Check sheet for the modelled part. Datum: model origin and axes. Units: mm. A direction names the side the tool comes from. Give positions to 0.01 mm unless a question says otherwise; leave off trailing zeros. Loops run counter-clockwise (first coordinate to the right, second up) from the corner with the lowest first, then second, coordinate; pieces in that order, holes last. Notation, with made-up numbers: (85.5, 7) - (127.5, 7) arc R20 ccw to (127.5, 46) - close; hole circle Ø10 at (-5, 69.5). An arc over 180 degrees is marked (long way). Use CSV: the item, a comma, the result in double quotes.
from build123d import *

# Parameters (mm, degrees)
F0_R           = 9.525
F1_DEPTH       = 38.1
F4_W           = 7.6494621422
F4_H           = 6.35
F5_DEPTH       = 12.7
F8_D           = 14.732
F8_DEPTH       = 69.85
F8_TIP         = 4.4259393198
F8_ON_F7_D     = 14.732
F8_ON_F7_DEPTH = 69.85
F8_ON_F7_TIP   = 4.4259393198
F9_T4_DEPTH    = 51.5282991577
F9_S5_R        = 9.525
F9_T6_DEPTH    = 28
F9_T10_DEPTH   = 51.965031671
F9_S11_R       = 9.525
F9_T12_DEPTH   = 28
F9_T16_DEPTH   = 51.965031671
F9_S17_R       = 9.525
F9_T18_DEPTH   = 28
F9_T22_DEPTH   = 51.5282991577
F9_S23_R       = 9.525
F9_T24_DEPTH   = 28


# Not quite as in the source:
# - a fillet or chamfer that OpenCascade refuses, or shapes differently, is made with other operations: its cross-section is extruded or revolved along the edge and cut away or added
# - a feature of the source that left no trace in its solid (it failed there, or was rolled back) is left out


with BuildPart() as f1:
    # F0 (on Top) → F1 (new body, symmetric)
    with BuildSketch(Plane.XY):
        with Locations((-15.875, 0)):
            Circle(F0_R)
    extrude(amount=F1_DEPTH, both=True)



with BuildPart() as f1b:
    # F0 (on Top) → F1, piece 2 (new body, symmetric)
    with BuildSketch(Plane.XY):
        with Locations((15.875, 0)):
            Circle(F0_R)
    extrude(amount=F1_DEPTH, both=True)


with BuildPart() as f1_1:
    add(f1.part)

    add(f1b.part)  # F5 merges F1b
    # F4 (on Top) → F5 (join, symmetric)
    with BuildSketch(Plane.XY):
        with Locations((-3.8247310711, 3.175)):
            Rectangle(F4_W, F4_H)
        Polygon((7.4973143637, 0), (0, 0), (0, -6.35), (7.6071062533, -6.35), align=None)
        Polygon((0, 6.35), (0, 0), (7.4973143637, 0), (7.6071062533, 6.35), align=None)
        with Locations((-3.8247310711, -3.175)):
            Rectangle(F4_W, F4_H)
    extrude(amount=F5_DEPTH, both=True)

    # F8
    with Locations(Plane.XY.offset(38.1)):
        with Locations((-15.875, 0)):
            Hole(F8_D / 2, depth=F8_DEPTH)
            with Locations((0, 0, -(F8_DEPTH + F8_TIP / 2))):  # 118° drill point
                Cone(0, F8_D / 2, F8_TIP, mode=Mode.SUBTRACT)

    # F8 on F7
    with Locations(Plane.XY.offset(38.1)):
        with Locations((15.875, 0)):
            Hole(F8_ON_F7_D / 2, depth=F8_ON_F7_DEPTH)
            with Locations((0, 0, -(F8_ON_F7_DEPTH + F8_ON_F7_TIP / 2))):  # 118° drill point
                Cone(0, F8_ON_F7_D / 2, F8_ON_F7_TIP, mode=Mode.SUBTRACT)

    # F9: chamfer of 5.08 on 4 edges, made by hand


with BuildPart() as f9_tool2:
    # F9_s3 → F9_t4 (new body)
    with BuildSketch(Plane.XY.offset(25.7641495789)):
        Polygon((-7.6494621422, -1.27), (-2.5694621422, -6.35), (-7.6494621422, -6.35), align=None)
    extrude(amount=-F9_T4_DEPTH)

    # F9_s5 → F9_t6 (cut, symmetric)
    with BuildSketch(Plane.XY):
        with Locations((-15.875, 0)):
            Circle(F9_S5_R)
    extrude(amount=F9_T6_DEPTH, both=True, mode=Mode.SUBTRACT)


with BuildPart() as f1_2:
    add(f1_1.part)

    # F9_t1: cut F9_tool2
    add(f9_tool2.part, mode=Mode.SUBTRACT)


with BuildPart() as f9_tool8:
    # F9_s9 → F9_t10 (new body)
    with BuildSketch(Plane.XY.offset(25.9825158355)):
        Polygon((7.5177543218, -1.1821796141), (2.438513475, -6.35), (7.6071062533, -6.35), align=None)
    extrude(amount=-F9_T10_DEPTH)

    # F9_s11 → F9_t12 (cut, symmetric)
    with BuildSketch(Plane.XY):
        with Locations((15.875, 0)):
            Circle(F9_S11_R)
    extrude(amount=F9_T12_DEPTH, both=True, mode=Mode.SUBTRACT)


with BuildPart() as f1_3:
    add(f1_2.part)

    # F9_t7: cut F9_tool8
    add(f9_tool8.part, mode=Mode.SUBTRACT)


with BuildPart() as f9_tool14:
    # F9_s15 → F9_t16 (new body)
    with BuildSketch(Plane.XY.offset(-25.9825158355)):
        Polygon((7.5177543218, 1.1821796141), (2.438513475, 6.35), (7.6071062533, 6.35), align=None)
    extrude(amount=F9_T16_DEPTH)

    # F9_s17 → F9_t18 (cut, symmetric)
    with BuildSketch(Plane.XY):
        with Locations((15.875, 0)):
            Circle(F9_S17_R)
    extrude(amount=F9_T18_DEPTH, both=True, mode=Mode.SUBTRACT)


with BuildPart() as f1_4:
    add(f1_3.part)

    # F9_t13: cut F9_tool14
    add(f9_tool14.part, mode=Mode.SUBTRACT)


with BuildPart() as f9_tool20:
    # F9_s21 → F9_t22 (new body)
    with BuildSketch(Plane.XY.offset(25.7641495789)):
        Polygon((-7.6494621422, 1.27), (-2.5694621422, 6.35), (-7.6494621422, 6.35), align=None)
    extrude(amount=-F9_T22_DEPTH)

    # F9_s23 → F9_t24 (cut, symmetric)
    with BuildSketch(Plane.XY):
        with Locations((-15.875, 0)):
            Circle(F9_S23_R)
    extrude(amount=F9_T24_DEPTH, both=True, mode=Mode.SUBTRACT)


with BuildPart() as f1_5:
    add(f1_4.part)

    # F9_t19: cut F9_tool20
    add(f9_tool20.part, mode=Mode.SUBTRACT)


solid = f1_5.part
1. Sectioned sample at B-B, the plane z = -30. Record the boundary of the cut face in (x, y) (3 decimals).
Completed:
outline,"circle Ø19.05 at (-15.875, 0); circle Ø19.05 at (15.875, 0); hole circle Ø14.732 at (-15.875, 0); hole circle Ø14.732 at (15.875, 0)"
2. Sectioned sample at D-D, the plane y = -4.75. State how many separate pieces and enclosed holes the cut face has, and give its area (3 significant figures).
Completed:
separate pieces,"3"
enclosed holes,"0"
area,"1,130 mm²"
3. Release check for a two-part mould opening along Y. For faces 4 (the face through (-17.15, 0.06, -35.41)), 5 (the face through (-6.79, 2.86, 0.53)), 6 (the face through (4.54, 4.21, -0.18)) record: released by +Y, released by -Y, zero draft, split by the parting line, or undercut.
Completed:
face 4,"undercut"
face 5,"split by the parting line"
face 6,"released by +Y"
4. Scan lines: line 1 along Y through (x, z) = (15.5, -4); line 2 along X through (y, z) = (-3, -31); line 3 along X through (y, z) = (2.5, -31.5). Record each from-to range of solid material in increasing order.
Completed:
line 1,"y = -9.52 to -7.36, 7.36 to 9.52"
line 2,"x = -24.92 to -22.6, -9.15 to -6.83, 6.83 to 9.15, 22.6 to 24.92"
line 3,"x = -25.07 to -22.8, -8.95 to -6.68, 6.68 to 8.95, 22.8 to 25.07"
5. Set-up check for faces 1 (the face through (0, 6.35, 0)), 2 (the face through (-10.03, -4.48, 2.69)), 3 (the face through (4.54, -4.21, 0.18)): record each of +Z, -Z, +X, -X, +Y, -Y from which the full face is reachable in a straight line by a thin tool's end or side.
Completed:
face 1,"+Z, -Z, +Y"
face 2,"+Z"
face 3,"+Z, -Z, -Y"
6. Sectioned sample at A-A, the plane z = 7.5. Record the boundary of the cut face in (x, y) (3 decimals).
Completed:
outline,"(-6.629, -2.29) - (-2.569, -6.35) - (2.439, -6.35) - (6.59, -2.126) arc R9.525 ccw (long way) to (6.59, 2.126) - (2.439, 6.35) - (-2.569, 6.35) - (-6.629, 2.29) arc R9.525 ccw (long way) to start; hole circle Ø14.732 at (-15.875, 0); hole circle Ø14.732 at (15.875, 0)"
7. Go/stop test with flat-tipped pins: pin 1 Ø4 at (x, y) = (-2, -2) entering from -Z; pin 2 Ø10 at (x, y) = (0.5, 3) entering from +Z; pin 3 Ø6 at (y, z) = (-7, 8.5) entering from -X; pin 4 Ø5 at (y, z) = (1.5, 5) entering from +X. Record where each tip stops, or that it passes through.
Completed:
pin 1,"stops at z = -12.7"
pin 2,"stops at z = 12.7"
pin 3,"stops at x = -24.52"
pin 4,"stops at x = 25.4"
8. Sectioned sample at C-C, the plane x = 1. Record the boundary of the cut face in (y, z), and give its area (3 significant figures).
Completed:
outline,"(-6.35, -12.7) - (6.35, -12.7) - (6.35, 12.7) - (-6.35, 12.7) - close"
area,"323 mm²"
